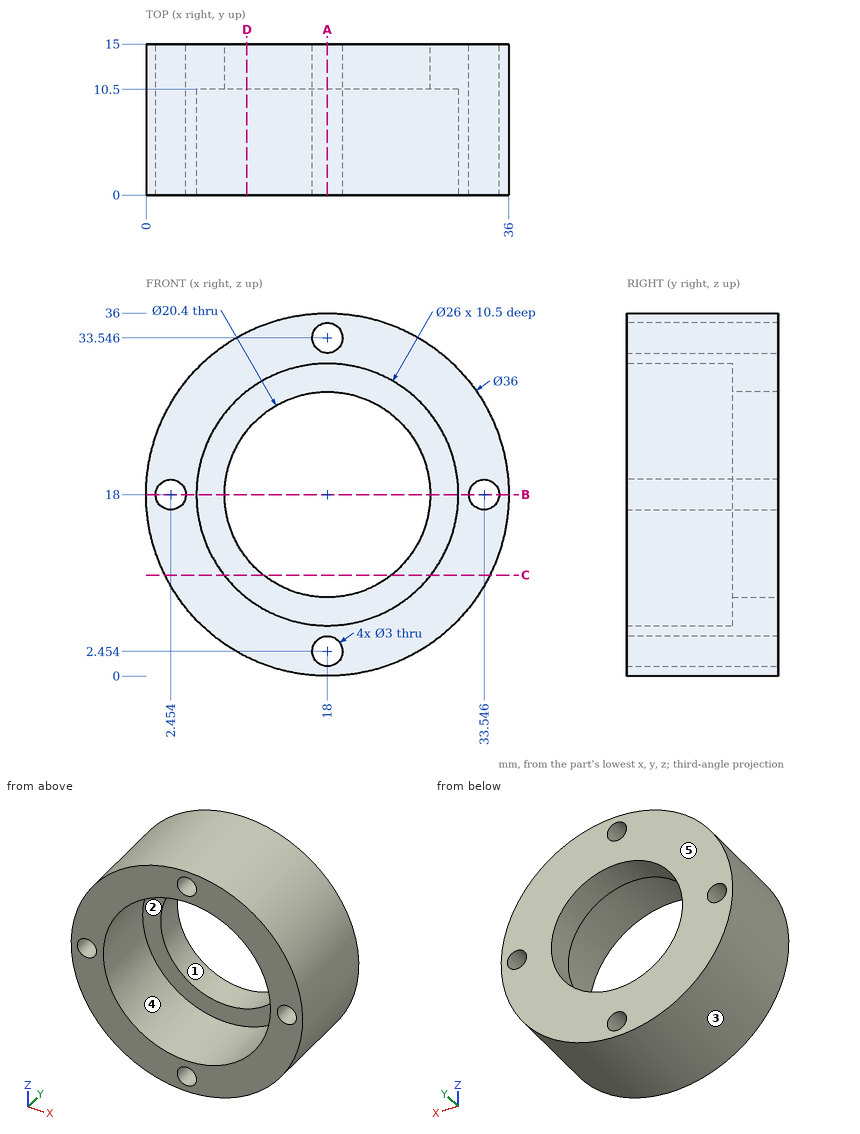
Check sheet for the drawn part. Datum: minimum x, y, z corner. Units: mm. A direction names the side the tool comes from. Coordinates: 2 decimals unless noted, no trailing zeros. Write each loop counter-clockwise with the first axis right and the second up, starting at its lowest first coordinate (ties: lowest second). Pieces come first, ordered by that corner, then holes. Notation, with made-up numbers: (21, 30.5) - (76, 30.5) arc R15 cw to (76, 40.5) - close; hole circle Ø3 at (-35, 49.25). An arc over 180 degrees is marked (long way). Answer as a JSON object with one key per item and string values.
(1) Gauge pin test, flat ends, axial feed: pin 1 Ø1.5 at (y, z) = (5, 30.5) entering from -X; pin 2 Ø3 at (y, z) = (10.5, 26) entering from +X; pin 3 Ø2 at (x, y) = (32, 8) entering from +Z. Record the tip position at first contact, or that the pin passes through.
Report:
{"pin 1": "x = 4.36", "pin 2": "x = 34.79", "pin 3": "z = 30.45"}
(2) Mould release check, pull along X, two halves, no side actions. Record for the marked faces 3, 4 and 5: pulls with the +X half, pulls with the -X half, needs draft (parallel to the pull), parting line crosses it, or undercut.
Report:
{"face 3": "parting line crosses it", "face 4": "undercut", "face 5": "needs draft"}
(3) Cross-section at A-A on x = 18. Record the cut outline in (y, z).
Report:
{"outline": "(0, 0) - (15, 0) - (15, 0.95) - (0, 0.95) - close; (0, 3.95) - (15, 3.95) - (15, 7.8) - (10.5, 7.8) - (10.5, 5) - (0, 5) - close; (0, 31) - (10.5, 31) - (10.5, 28.2) - (15, 28.2) - (15, 32.05) - (0, 32.05) - close; (0, 35.05) - (15, 35.05) - (15, 36) - (0, 36) - close"}
(4) Cross-section at D-D on x = 10. Record the cut outline in (y, z).
Report:
{"outline": "(0, 1.88) - (15, 1.88) - (15, 11.67) - (10.5, 11.67) - (10.5, 7.75) - (0, 7.75) - close; (0, 28.25) - (10.5, 28.25) - (10.5, 24.33) - (15, 24.33) - (15, 34.12) - (0, 34.12) - close"}
(5) Thickness scan on line 1 along X through (y, z) = (6.5, 18); line 2 along Y through (x, z) = (29, 17.5); line 3 along Z through (x, y) = (25, 4.75) (1 decimal). Record the ranges inside material, lowest first.
Report:
{"line 1": "0 to 0.95, 3.95 to 5, 31 to 32.05, 35.05 to 36", "line 2": "10.5 to 15", "line 3": "1.4 to 7, 29 to 34.6"}
(6) Cross-section at B-B on z = 18. Record the cut outline in (x, y), plus the area to 3 significant figures.
Report:
{"outline": "(0, 0) - (0.95, 0) - (0.95, 15) - (0, 15) - close; (3.95, 0) - (5, 0) - (5, 10.5) - (7.8, 10.5) - (7.8, 15) - (3.95, 15) - close; (28.2, 10.5) - (31, 10.5) - (31, 0) - (32.05, 0) - (32.05, 15) - (28.2, 15) - close; (35.05, 0) - (36, 0) - (36, 15) - (35.05, 15) - close", "area": "85.2 mm^2"}
(7) Cross-section at C-C on z = 10. Record the cut outline in (x, y).
Report:
{"outline": "(1.88, 0) - (7.75, 0) - (7.75, 10.5) - (11.67, 10.5) - (11.67, 15) - (1.88, 15) - close; (24.33, 10.5) - (28.25, 10.5) - (28.25, 0) - (34.12, 0) - (34.12, 15) - (24.33, 15) - close"}
(8) Tool access check on the marked faces 1 and 2. Record the directions out of +Z, -Z, +X, -X, +Y, -Y that give a thin tool (end or side, any length) a straight path to the whole face; none if there is none.
Report:
{"face 1": "+Y, -Y", "face 2": "-Y"}
